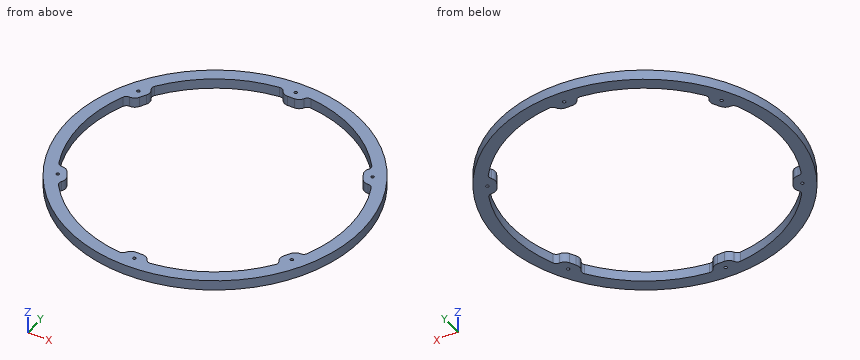
```python
from build123d import *

# Parameters (mm, degrees)
SKETCH1_R           = 147.5
SKETCH1_R_2         = 135
BOSS_EXTRUDE1_DEPTH = 10
BOSS_EXTRUDE2_START = -10
BOSS_EXTRUDE2_DEPTH = 10
FILLET1_R           = 5
FILLET2_R           = 8
CUT_EXTRUDE1_REACH  = 210.836
SKETCH5_R           = 1.5
CIRPATTERN1_DEPTH   = 10
CIRPATTERN1_2_DEPTH = 10


# Read off the part's stored shape, not the designer's step: CirPattern1
with BuildPart() as part:
    # Sketch1 → Boss-Extrude1 (new body)
    with BuildSketch(Plane.XY):
        Circle(SKETCH1_R)
        Circle(SKETCH1_R_2, mode=Mode.SUBTRACT)
    extrude(amount=BOSS_EXTRUDE1_DEPTH)

    # Sketch3 → Boss-Extrude2 (add)
    with BuildSketch(Plane.XY.offset(10).offset(BOSS_EXTRUDE2_START)):
        with BuildLine():
            Line((-10, 127), (10, 127))
            Line((10, 127), (10, 134.629120178))
            ThreePointArc((10, 134.629120178), (0, 135), (-10, 134.629120178))
            Line((-10, 134.629120178), (-10, 127))
        make_face()
    extrude(amount=BOSS_EXTRUDE2_DEPTH)

    # Fillet1
    fillet1_edges = [part.edges().sort_by_distance(p)[0] for p in [
        (-10, 134.629120178, 5),
        (10, 134.629120178, 5),
    ]]
    fillet(fillet1_edges, radius=FILLET1_R)

    # Fillet2
    fillet2_edges = [part.edges().sort_by_distance(p)[0] for p in [
        (10, 127, 5),
        (-10, 127, 5),
    ]]
    fillet(fillet2_edges, radius=FILLET2_R)

    # Sketch5 → Cut-Extrude1 (cut, up to next)
    with BuildSketch(Plane.XY.offset(10), mode=Mode.PRIVATE) as cut_extrude1_sk1:
        with Locations((0, 135)):
            Circle(SKETCH5_R)
    cut_extrude1_tool1 = extrude(cut_extrude1_sk1.sketch, amount=-CUT_EXTRUDE1_REACH, mode=Mode.PRIVATE) & part.part
    add(cut_extrude1_tool1.solids().sort_by_distance((0, 135, 10))[0], mode=Mode.SUBTRACT)

    # CirPattern1 outline → CirPattern1 (cut)
    with BuildSketch(Plane.XY):
        with BuildLine():
            ThreePointArc((-116.156224207, 68.794851392), (-118.212467617, 68.25), (-117.656201059, 66.196815275))
            ThreePointArc((-117.656201059, 66.196815275), (-116.913429511, 67.5), (-116.156224207, 68.794851392))
        make_face()
        with BuildLine():
            ThreePointArc((-116.156224207, -68.794851392), (-116.913429511, -67.5), (-117.656201059, -66.196815275))
            ThreePointArc((-117.656201059, -66.196815275), (-118.212467617, -68.25), (-116.156224207, -68.794851392))
        make_face()
        with BuildLine():
            ThreePointArc((1.499976852, -134.991666667), (0, -135), (-1.499976852, -134.991666667))
            ThreePointArc((-1.499976852, -134.991666667), (0, -136.5), (1.499976852, -134.991666667))
        make_face()
        with BuildLine():
            ThreePointArc((117.656201059, -66.196815275), (116.913429511, -67.5), (116.156224207, -68.794851392))
            ThreePointArc((116.156224207, -68.794851392), (118.212467617, -68.25), (117.656201059, -66.196815275))
        make_face()
        with BuildLine():
            ThreePointArc((116.156224207, 68.794851392), (116.913429511, 67.5), (117.656201059, 66.196815275))
            ThreePointArc((117.656201059, 66.196815275), (118.212467617, 68.25), (116.156224207, 68.794851392))
        make_face()
    extrude(amount=CIRPATTERN1_DEPTH, mode=Mode.SUBTRACT)

    # CirPattern1 2 outline → CirPattern1 2 (add)
    with BuildSketch(Plane.XY):
        with BuildLine():
            ThreePointArc((-119.055197564, 56.567845161), (-114.80628077, 57.519573858), (-111.685156467, 60.555634549))
            Line((-111.685156467, 60.555634549), (-108.285296095, 66.444365451))
            ThreePointArc((-108.285296095, 66.444365451), (-107.216552561, 70.665368732), (-108.516789729, 74.820902963))
            ThreePointArc((-108.516789729, 74.820902963), (-109.329067487, 77.707176829), (-108.344090318, 80.539171173))
            ThreePointArc((-108.344090318, 80.539171173), (-112.403647927, 74.76911082), (-116.156224207, 68.794851392))
            ThreePointArc((-116.156224207, 68.794851392), (-115.614391405, 66.75), (-117.656201059, 66.196815275))
            ThreePointArc((-117.656201059, 66.196815275), (-120.953773352, 59.959859172), (-123.921013395, 53.559148978))
            ThreePointArc((-123.921013395, 53.559148978), (-121.960922934, 55.828161401), (-119.055197564, 56.567845161))
        make_face()
        with BuildLine():
            ThreePointArc((119.055197564, 56.567845161), (121.960922934, 55.828161401), (123.921013394, 53.559148978))
            ThreePointArc((123.921013394, 53.559148978), (120.953773352, 59.959859172), (117.656201059, 66.196815275))
            ThreePointArc((117.656201059, 66.196815275), (115.614391405, 66.75), (116.156224207, 68.794851392))
            ThreePointArc((116.156224207, 68.794851392), (112.403647927, 74.76911082), (108.344090318, 80.539171173))
            ThreePointArc((108.344090318, 80.539171173), (109.329067487, 77.707176829), (108.516789729, 74.820902963))
            ThreePointArc((108.516789729, 74.820902963), (107.216552561, 70.665368732), (108.285296095, 66.444365451))
            Line((108.285296095, 66.444365451), (111.685156467, 60.555634549))
            ThreePointArc((111.685156467, 60.555634549), (114.80628077, 57.519573858), (119.055197564, 56.567845161))
        make_face()
        with BuildLine():
            ThreePointArc((108.516789729, -74.820902963), (109.329067487, -77.707176829), (108.344090318, -80.539171173))
            ThreePointArc((108.344090318, -80.539171173), (112.403647927, -74.76911082), (116.156224207, -68.794851392))
            ThreePointArc((116.156224207, -68.794851392), (115.614391405, -66.75), (117.656201059, -66.196815275))
            ThreePointArc((117.656201059, -66.196815275), (120.953773352, -59.959859172), (123.921013395, -53.559148978))
            ThreePointArc((123.921013395, -53.559148978), (121.960922934, -55.828161401), (119.055197564, -56.567845161))
            ThreePointArc((119.055197564, -56.567845161), (114.80628077, -57.519573858), (111.685156467, -60.555634549))
            Line((111.685156467, -60.555634549), (108.285296095, -66.444365451))
            ThreePointArc((108.285296095, -66.444365451), (107.216552561, -70.665368732), (108.516789729, -74.820902963))
        make_face()
        with BuildLine():
            ThreePointArc((-10.538407835, -131.388748124), (-12.631855447, -133.53533823), (-15.576923077, -134.098320152))
            ThreePointArc((-15.576923077, -134.098320152), (-8.550125426, -134.728969992), (-1.499976852, -134.991666667))
            ThreePointArc((-1.499976852, -134.991666667), (0, -133.5), (1.499976852, -134.991666667))
            ThreePointArc((1.499976852, -134.991666667), (8.550125426, -134.728969992), (15.576923077, -134.098320152))
            ThreePointArc((15.576923077, -134.098320152), (12.631855447, -133.53533823), (10.538407835, -131.388748124))
            ThreePointArc((10.538407835, -131.388748124), (7.589728209, -128.18494259), (3.399860372, -127))
            Line((3.399860372, -127), (-3.399860372, -127))
            ThreePointArc((-3.399860372, -127), (-7.589728209, -128.18494259), (-10.538407835, -131.388748124))
        make_face()
        with BuildLine():
            ThreePointArc((-119.055197564, -56.567845161), (-121.960922934, -55.828161401), (-123.921013394, -53.559148978))
            ThreePointArc((-123.921013394, -53.559148978), (-120.953773352, -59.959859172), (-117.656201059, -66.196815275))
            ThreePointArc((-117.656201059, -66.196815275), (-115.614391405, -66.75), (-116.156224207, -68.794851392))
            ThreePointArc((-116.156224207, -68.794851392), (-112.403647927, -74.76911082), (-108.344090318, -80.539171173))
            ThreePointArc((-108.344090318, -80.539171173), (-109.329067487, -77.707176829), (-108.516789729, -74.820902963))
            ThreePointArc((-108.516789729, -74.820902963), (-107.216552561, -70.665368732), (-108.285296095, -66.444365451))
            Line((-108.285296095, -66.444365451), (-111.685156467, -60.555634549))
            ThreePointArc((-111.685156467, -60.555634549), (-114.80628077, -57.519573858), (-119.055197564, -56.567845161))
        make_face()
    extrude(amount=CIRPATTERN1_2_DEPTH)


solid = part.part
```
Part model, mm, in its own coordinate system. Round coordinates to 2 decimals unless told otherwise and drop trailing zeros. Loops run counter-clockwise (first coordinate to the right, second up) from the corner with the lowest first, then second, coordinate; pieces in that order, holes last.
Item 1: Cut at A-A, the plane y = 0. Give the cut face in (x, z).
Item 2: Cut at B-B, the plane x = 23.5. Give the cut face in (y, z), then the cut area to 3 significant figures.
Item 3: Drill centre lines: line 1 (Y direction, x = 99.5, z = 2.5); line 2 (X direction, y = 4, z = 8.5); line 3 (Y direction, x = -117, z = 8.5). Where is each one in solid material? Low to high.
Item 4: Cut at C-C, the plane z = 7.5. State how many separate pieces and enclosed holes the cut face has, then the cut area to 3 significant figures.
Item 5: Drop flat-ended pins along their axis: P1, Ø1, axis at x = -16, z = 8, coming from the +Y side; P2, Ø4, axis at x = -56, z = 2.5, coming from the -Y side; P3, Ø4, axis at x = -66, z = 6, coming from the +Y side. Give the stop position or say it passes through.
A:
1. outline: (-147.5, 0) - (-135, 0) - (-135, 10) - (-147.5, 10) - close; (135, 0) - (147.5, 0) - (147.5, 10) - (135, 10) - close
2. outline: (-145.62, 0) - (-132.94, 0) - (-132.94, 10) - (-145.62, 10) - close; (132.94, 0) - (145.62, 0) - (145.62, 10) - (132.94, 10) - close
2. area: 254 mm2
3. line 1: y = -108.89 to -91.24, 91.24 to 108.89
3. line 2: x = -147.45 to -134.94, 134.94 to 147.45
3. line 3: y = -89.82 to -69, -66 to -56.72, 56.72 to 66, 69 to 89.82
4. separate pieces: 1
4. enclosed holes: 7
4. area: 12,000 mm2
5. P1: stops at y = 146.68
5. P2: stops at y = -137.26
5. P3: stops at y = 132.89
